Can you work these out from the model? Positions are in its coordinate system, mm. Give positions to 0.01 mm unless a question says otherwise; leave off trailing zeros. Order: outer loops, then holes, each group sorted by start corner. A loop starts at its lowest first (then second) coordinate and runs counter-clockwise, first axis right, second up. Notation, with made-up numbers: (-30, 63) - (-15, 63) arc R26 cw to (-15, 86) - close; hole circle Ø4 at (-34, 26). An arc over 180 degrees is marked (long way). Write each question's results on one line, items separated by ' | '. Start each with the question number.
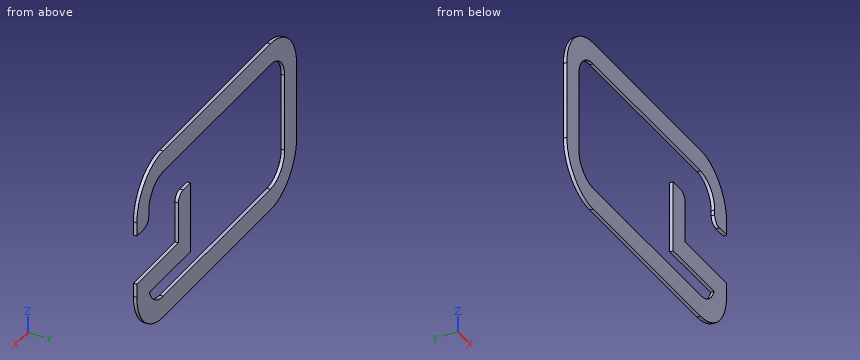
from build123d import *

# Parameters (mm, degrees)
BOSS_EXTRUDE1_DEPTH = 4


with BuildPart() as part:
    # Sketch1 → Boss-Extrude1 (new body)
    with BuildSketch(Plane(origin=(0, 0, 0), x_dir=(1, 0, 0), z_dir=(0, 1, 0))):
        with BuildLine():
            Line((223, 154), (223, 71))
            Line((223, 71), (238, 71))
            ThreePointArc((238, 71), (245.071067812, 73.928932188), (248, 81))
            Line((248, 81), (248, 129))
            Line((248, 129), (335, 129))
            Line((335, 129), (335, 145))
            ThreePointArc((335, 145), (318.890872965, 183.890872965), (280, 200))
            Line((280, 200), (55, 200))
            ThreePointArc((55, 200), (16.109127035, 183.890872965), (0, 145))
            Line((0, 145), (0, 55))
            ThreePointArc((0, 55), (16.109127035, 16.109127035), (55, 0))
            Line((55, 0), (280, 0))
            ThreePointArc((280, 0), (318.890872965, 16.109127035), (335, 55))
            Line((335, 55), (335, 71))
            Line((335, 71), (320, 71))
            ThreePointArc((320, 71), (312.928932188, 68.071067812), (310, 61))
            Line((310, 61), (310, 55))
            ThreePointArc((310, 55), (301.213203436, 33.786796564), (280, 25))
            Line((280, 25), (55, 25))
            ThreePointArc((55, 25), (33.786796564, 33.786796564), (25, 55))
            Line((25, 55), (25, 145))
            ThreePointArc((25, 145), (33.786796564, 166.213203436), (55, 175))
            Line((55, 175), (280, 175))
            ThreePointArc((280, 175), (297.748239349, 169.186773245), (308.618176043, 154))
            Line((308.618176043, 154), (223, 154))
        make_face()
    extrude(amount=BOSS_EXTRUDE1_DEPTH)


solid = part.part
Q1. If I drill on probe 1 along Z at (x, y) = (251, 2.5); probe 2 along X at (y, z) = (2.7, -94); probe 3 along X at (y, z) = (1.15, -146), over which ranges is the centre line in solid material (lowest first)? Write a range as from..to.
Q2. Will these pins go through, and if not, where does the flat tip stop? P1, Ø1.2, axis at y = 3, z = -98.5, coming from the +X side; P2, Ø1.5, axis at y = 3, z = -167.5, coming from the -X side.
Q3. If we section it at C-C (x = 118): Please give me the cut outline in (y, z).
Q4. If we section it at A-A (z = -97): Please give me the cut outline in (x, y), plus the area to 3 significant figures.
Q5. If we section it at B-B (x = 264): Please give me the cut outline in (y, z).
Q6. If we section it at D-D (y = 1.1): Please give me the cut outline in (x, z).
Findings below:
1) probe 1: z = -200..-175, -154..-129, -25..0 | probe 2: x = 0..25, 223..248 | probe 3: x = 0.01..25.02, 223..334.99
2) P1: stops at x = 248 | P2: stops at x = 4.48
3) outline: (0, -200) - (4, -200) - (4, -175) - (0, -175) - close; (0, -25) - (4, -25) - (4, 0) - (0, 0) - close
4) outline: (0, 0) - (25, 0) - (25, 4) - (0, 4) - close; (223, 0) - (248, 0) - (248, 4) - (223, 4) - close | area: 200 mm2
5) outline: (0, -200) - (4, -200) - (4, -175) - (0, -175) - close; (0, -154) - (4, -154) - (4, -129) - (0, -129) - close; (0, -25) - (4, -25) - (4, 0) - (0, 0) - close
6) outline: (0, -145) arc R55 ccw to (55, -200) - (280, -200) arc R55 ccw to (335, -145) - (335, -129) - (248, -129) - (248, -81) arc R10 ccw to (238, -71) - (223, -71) - (223, -154) - (308.62, -154) arc R30 cw to (280, -175) - (55, -175) arc R30 cw to (25, -145) - (25, -55) arc R30 cw to (55, -25) - (280, -25) arc R30 cw to (310, -55) - (310, -61) arc R10 ccw to (320, -71) - (335, -71) - (335, -55) arc R55 ccw to (280, 0) - (55, 0) arc R55 ccw to (0, -55) - close
